Autodesk Inventor part; units mm, degrees
ref_plane "YZ Plane" through (0, 0, 0) normal (1, 0, 0) x (0, 1, 0)
ref_plane "XZ Plane" through (0, 0, 0) normal (0, 1, 0) x (-1, 0, 0)
ref_plane "XY Plane" through (0, 0, 0) normal (0, 0, 1) x (1, 0, 0)
sketch "Sketch1" plane through (0, 0, 0) normal (0, 0, 1) x (1, 0, 0)
  line L0 (49.2125, 0) -> (54.6328, 0)
  line L1 (357.1875, 0) -> (350.9902, 0)
  arc A0 (0, 49.2125) -> (65.0875, 2.6308) centre (49.2125, 49.2125) ccw
  arc A1 (345.2239, 1.4763) -> (406.4, 49.2125) centre (357.1875, 49.2125) ccw
  arc A2 (203.2, 19.05) -> (54.6328, 0) centre (202.8115, -566.7686) ccw
  arc A3 (350.9902, 0) -> (345.2239, 1.4763) centre (202.8115, -566.7686) ccw
  arc A4 (65.0875, 2.6308) -> (54.6328, 0) centre (202.8115, -566.7686) ccw
  arc A5 (350.9902, 0) -> (203.2, 19.05) centre (202.8115, -566.7686) ccw
  line L2 (0, 49.2125) -> (0, 228.6)
  line L3 (406.4, 228.6) -> (406.4, 49.2125)
  line L4 (0, 228.6) -> (406.4, 228.6)
  point P0 (0, 0)
  point P1 (57.0671, 0.6309)
extrude "Extrusion1" add sketch "Sketch1" along normal blind 5.5563 contours A0 L2 L4 L3 A1 A5 A2
sketch "Sketch5" plane through (0, 0, 5.5563) normal (0, 0, 1) x (1, 0, 0)
  line L0 (128.7512, 178.3406) -> (279.9627, 178.3406) construction
  line L1 (279.9627, 178.3406) -> (279.9627, 123.3225) construction
  line L2 (279.9627, 123.3225) -> (128.7512, 123.3225) construction
  line L3 (128.7512, 123.3225) -> (128.7512, 178.3406) construction
  point P0 (0, 0)
sketch "Sketch6" plane through (0, 0, 5.5563) normal (0, 0, 1) x (1, 0, 0)
  line L0 (406.4, 228.6) -> (0, 228.6)
  line L1 (0, 228.6) -> (0, 49.2125)
  circle A0 centre (31.75, 196.85) radius 2.9337
  line L2 (406.4, 49.2125) -> (406.4, 228.6)
  circle A1 centre (374.65, 196.85) radius 2.9337
  circle A2 centre (203.2, 196.85) radius 2.9337
  arc A3 (345.2239, 1.4763) -> (406.4, 49.2125) centre (357.1875, 49.2125) ccw
  circle A4 centre (361.7391, 44.6609) radius 2.9337
  arc A5 (0, 49.2125) -> (57.0671, 0.6309) centre (49.2125, 49.2125) ccw
  circle A6 centre (44.6609, 44.6609) radius 2.9337
  point P0 (0, 0)
  point P1 (0, 0)
extrude "Extrusion6" cut sketch "Sketch6" against normal up to surface (5.5563 mm away)
sketch "Sketch7" plane through (0, 0, 5.5563) normal (0, 0, 1) x (1, 0, 0)
  ellipse E0 centre (293.3334, 94.2801) end of major axis (293.3295, 96.2801) minor radius 2
  ellipse E1 centre (293.3643, 62.2802) end of major axis (293.3569, 64.2802) minor radius 2
  circle A0 centre (361.7412, 44.6631) radius 2.9337
  line L0 (361.7412, 44.6631) -> (293.3643, 44.6631)
  line L1 (293.3643, 44.6631) -> (293.3643, 62.2802)
  ellipse E2 centre (113.007, 94.278) end of major axis (113.0032, 96.278) minor radius 2
  ellipse E3 centre (113.0379, 62.2781) end of major axis (113.0305, 64.2781) minor radius 2
  line L2 (113.0379, 44.6609) -> (113.0379, 62.2781)
  circle A1 centre (293.3643, 78.2802) radius 4.699
  circle A2 centre (113.0379, 78.278) radius 4.699
  circle A3 centre (44.6609, 44.6609) radius 2.9337
  line L3 (44.6609, 44.6609) -> (113.0379, 44.6609)
  point P0 (0, 0)
  point P1 (0, 0)
  dimension "d59" = 17.6171
  dimension "d60" = 68.3769
  dimension "d61" = 17.6171
  dimension "d62" = 9.398
  dimension "d63" = 9.398
  dimension "d64" = 68.3769
extrude "Extrusion7" cut sketch "Sketch7" against normal through all contours E0 | E1 | E2 | E3
sketch "Sketch8" plane through (0, 0, 5.5563) normal (0, 0, 1) x (1, 0, 0)
  ellipse E0 centre (309.3078, 127.6497) end of major axis (309.3104, 126.2971) minor radius 1.3525
  ellipse E1 centre (277.3079, 127.5882) end of major axis (277.3105, 126.2356) minor radius 1.3525
  ellipse E2 centre (293.3334, 94.2801) end of major axis (293.3295, 96.2801) minor radius 2
  ellipse E3 centre (293.3334, 94.2801) end of major axis (293.3295, 96.2801) minor radius 2
  ellipse E4 centre (128.9815, 127.6475) end of major axis (128.9841, 126.295) minor radius 1.3525
  ellipse E5 centre (96.9816, 127.586) end of major axis (96.9842, 126.2335) minor radius 1.3525
  ellipse E6 centre (113.007, 94.278) end of major axis (113.0032, 96.278) minor radius 2
  ellipse E7 centre (113.007, 94.278) end of major axis (113.0032, 96.278) minor radius 2
  point P0 (0, 0)
extrude "Extrusion8" cut sketch "Sketch8" against normal through all contours E0 | E1 | E4 | E5
properties part number "FTC Outside Panels" material "Wood (Oak)"
Design review of the part built by this model. Coordinates are the model's own, in mm. Give positions to 0.01 mm unless a question says otherwise; leave off trailing zeros. Order: outer loops, then holes, each group sorted by start corner. A loop starts at its lowest first (then second) coordinate and runs counter-clockwise, first axis right, second up. Notation, with made-up numbers: (58.5, 4) -> (107.5, 4) arc R37 cw to (107.5, 42) -> close; hole circle Ø3 at (-15.5, -5). An arc over 180 degrees is marked (long way). Write item = value, one per line. Start each with the question number.
(1) We need section B-B on x = 85. Write out the cut boundary in (y, z).
(2) Mouldability with a two-part tool opening along X and no side actions: class faces 1 (the face through (200, 116, 5.556)), 2 (the face through (273.75, 14.74, 2.74)), 3 (the face through (128.53, 14.32, 2.74)) as +X half, -X half, draft (parallel to the pull), parting line (faces both ways), or undercut.
(3) We need section C-C on x = 222. Write out the cut boundary in (y, z), plus the area to 3 significant figures.
(4) We need section A-A on z = 2.45. State how many separate pieces and enclosed holes the cut face has, plus the area to 3 significant figures.
(5) To check wall thickness, follow line 1 along X through (y, z) = (196.85, 2.85); line 2 along Y through (x, z) = (292, 3.5); line 3 along Y through (x, z) = (31.75, 3.2). State the ranges of each line that lie inside material, in increasing order.
(6) For pin 1 (3.5 mm diameter, centred on x = 374.65, y = 196.85, fed in from +Z), flat-tipped, find the tip position at first contact; note if it passes through.
Numbers:
q1.outline = (7.08, 0) -> (228.6, 0) -> (228.6, 5.56) -> (7.08, 5.56) -> close
q2.face_1 = draft
q2.face_2 = undercut
q2.face_3 = undercut
q3.outline = (18.74, 0) -> (228.6, 0) -> (228.6, 5.56) -> (18.74, 5.56) -> close
q3.area = 1,170 mm^2
q4.separate_pieces = 1
q4.enclosed_holes = 13
q4.area = 87,900 mm^2
q5.line_1 = 0 to 28.82, 34.68 to 200.27, 206.13 to 371.72, 377.58 to 406.4
q5.line_2 = 12.22 to 60.82, 63.74 to 92.79, 95.77 to 228.6
q5.line_3 = 3.2 to 193.92, 199.78 to 228.6
q6.pin_1 = through
